Input: dimensioned drawing with shaded views. Units: mm. Origin: part minimum x, y, z. Round coordinates to 2 decimals unless told otherwise and drop trailing zeros. Loops run counter-clockwise (first coordinate to the right, second up) from the corner with the lowest first, then second, coordinate; pieces in that order, holes last.
Item 1: First-contact query: P1, Ø3, axis at x = 5.5, z = 24.5, coming from the -Y side; P2, Ø1, axis at x = 1.5, z = 10, coming from the -Y side; P3, Ø6, axis at x = 7.5, y = 12, coming from the -Z side. Flat tips, straight axial feed; report the tip coordinate or a pass-through.
Item 2: Pull-direction query (Y, two-part tool) for the marked faces 1, 2 and 3; classes: released by +Y, released by -Y, zero draft, split by the parting line, or undercut.
Item 3: Section query B-B on z = 25. Return loops of the section in (x, y).
Item 4: Ray query, L1, parallel to Z at x = 7.75, y = 24.5 (1 decimal); L2, parallel to Y at x = 6.25, z = 25; L3, parallel to Z at x = 8.25, y = 35.5. Return the intervals inside material, ascending.
Item 5: Section query C-C on x = 11.25. Return loops of the section in (y, z).
Item 6: Section query A-A on y = 25. Return loops of the section in (x, z), then the cut area to 3 significant figures.
Item 7: Section query D-D on y = 45. Return loops of the section in (x, z).
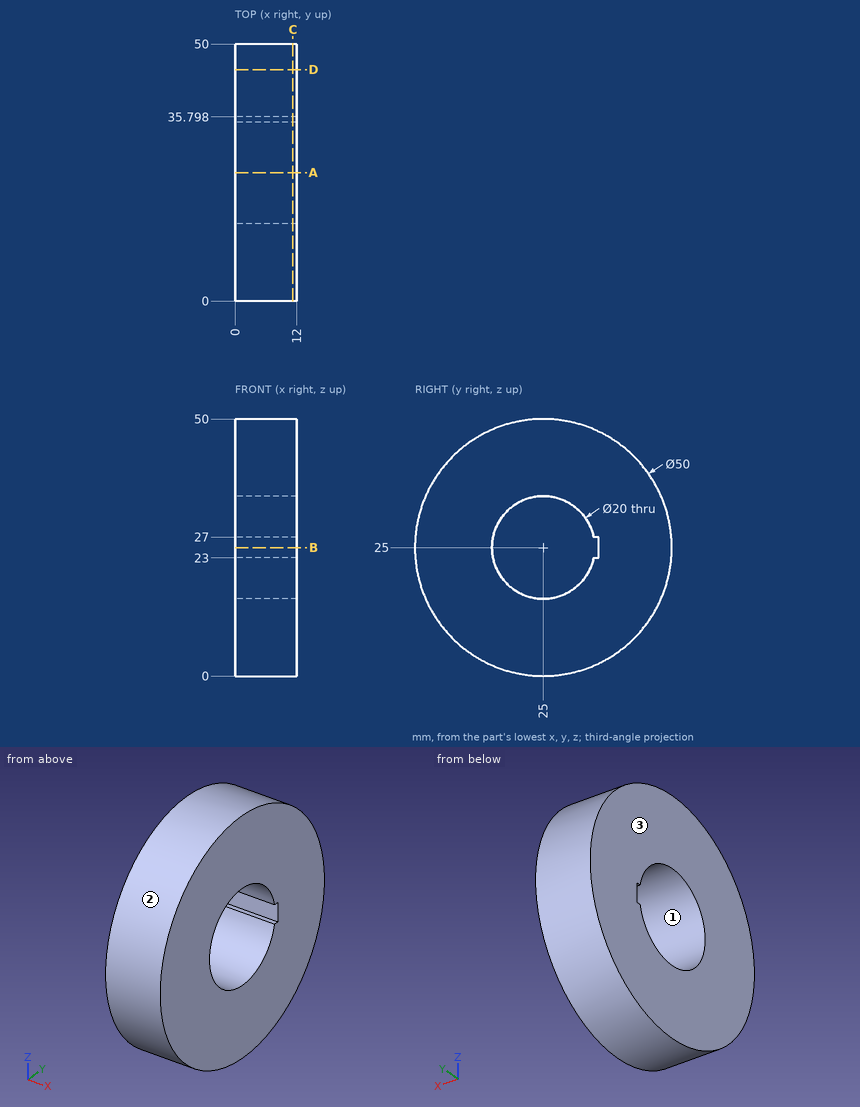
Data:
1. P1: stops at y = 0
1. P2: stops at y = 4.63
1. P3: stops at z = 2.09
2. face 1: undercut
2. face 2: split by the parting line
2. face 3: zero draft
3. outline: (0, 0) - (12, 0) - (12, 15) - (0, 15) - close; (0, 35.8) - (12, 35.8) - (12, 50) - (0, 50) - close
4. L1: z = 0 to 15, 35 to 50
4. L2: y = 0 to 15, 35.8 to 50
4. L3: z = 2.31 to 23, 27 to 47.69
5. outline: circle Ø50 at (25, 25); hole (34.8, 23) - (35.8, 23) - (35.8, 27) - (34.8, 27) arc R10 ccw (long way) to start
6. outline: (0, 0) - (12, 0) - (12, 15) - (0, 15) - close; (0, 35) - (12, 35) - (12, 50) - (0, 50) - close
6. area: 360 mm2
7. outline: (0, 10) - (12, 10) - (12, 40) - (0, 40) - close
